Work out the finished part from the listing and answer in its coordinate system (mm). Face numbers are marked on the shaded views. A direction names the side the tool comes from. Coordinates: 2 decimals unless noted, no trailing zeros. Order: outer loops, then holes, each group sorted by start corner. A loop starts at its lowest first (then second) coordinate and runs counter-clockwise, first axis right, second up. Notation, with made-up numbers: (-9, 1) -> (9, 1) arc R32 cw to (9, 29) -> close; hole circle Ø11 at (-18.75, -0.75). An arc over 180 degrees is marked (long way). Answer as CSV lines item,"result". Start each with the question number.
Item 1: A straight line is drawn through the part: L1, parallel to X at y = 12, z = 96 (3 decimals). Find the intervals that lie inside material, in ascending order.
Item 2: Section D-D (y = 45) is taken. Write down the section's boundary in (x, z) (3 decimals).
Item 3: Section A-A (y = 19.05) is taken. Write down the section's boundary in (x, z) (1 decimal).
Item 4: Section C-C (z = 145) is taken. Write down the section's boundary in (x, y) (3 decimals), then the cut area to 3 significant figures.
Item 5: Each of these flat-tipped pins is pushed along its axis until it touches: pin 1 Ø2 at (y, z) = (45, 113.5) entering from +X (3 decimals); pin 2 Ø2.5 at (x, y) = (15, 2) entering from -Z (3 decimals); pin 3 Ø1.6 at (x, z) = (1, 467.5) entering from -Y (3 decimals); pin 4 Ø12 at (x, y) = (11.5, 39) entering from +Z. Where does it stop, or does it pass through?
Item 6: Section B-B (x = 8.5) is taken. Write down the section's boundary in (y, z) (3 decimals).
Item 7: Which of the six approach directions +Z, -Z, +X, -X, +Y, -Y give full straight-line access (tool end or side, diameter ignored) to the marked faces 1 and 2?
Autodesk Inventor part; units mm, degrees
ref_plane "YZ Plane" through (0, 0, 0) normal (1, 0, 0) x (0, 1, 0)
ref_plane "XZ Plane" through (0, 0, 0) normal (0, 1, 0) x (-1, 0, 0)
ref_plane "XY Plane" through (0, 0, 0) normal (0, 0, 1) x (1, 0, 0)
sketch "Sketch1" plane through (0, 0, 0) normal (0, 0, 1) x (1, 0, 0)
  line L0 (0, 0) -> (25.4, 0)
  line L1 (25.4, 0) -> (25.4, 3.175)
  line L2 (3.175, 50.8) -> (0, 50.8)
  line L3 (0, 50.8) -> (0, 0)
  line L4 (3.175, 50.8) -> (3.175, 3.175)
  line L5 (3.175, 3.175) -> (25.4, 3.175)
  dimension "d0" = 50.8
  dimension "d1" = 25.4
  dimension "d2" = 3.175
  dimension "d3" = 3.175
extrude "Extrusion1" add sketch "Sketch1" along normal blind 482.6
sketch "Sketch2" plane through (0, 0, 0) normal (-1, 0, 0) x (0, 0, 1)
  line L0 (482.6, 0) -> (482.6, 50.8)
  line L1 (0, 0) -> (482.6, 0)
  circle A0 centre (466.725, 19.05) radius 11.1125
  dimension "d6" = 22.225
  dimension "d7" = 19.05
  dimension "d8" = 15.875
extrude "Extrusion2" cut sketch "Sketch2" against normal blind 508
sketch "Sketch3" plane through (0, 0, 0) normal (0, -1, 0) x (1, 0, 0)
  line L0 (0, 0) -> (0, 482.6)
  line L1 (0, 0) -> (25.4, 0)
  line L2 (25.4, 0) -> (25.4, 482.6)
  line L3 (0, 22.225) -> (25.4, 22.225)
  line L4 (25.4, 482.6) -> (0, 482.6)
  line L5 (0, 460.375) -> (25.4, 460.375)
  dimension "d13" = 22.225
  dimension "d16" = 22.225
extrude "Extrusion3" cut sketch "Sketch3" against normal blind 3.175 contours L0 L3 L2 L1 | L0 L4 L2 L5
equation "\"d3\" = d2"
equation "\"d16\" = d13"
properties part number "manipulator L frame right"
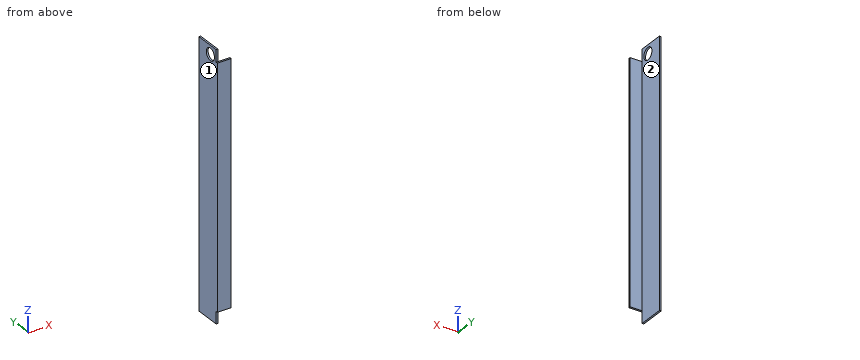
Checked values:
1,L1,"x = 0 to 3.175"
2,outline,"(0, 0) -> (3.175, 0) -> (3.175, 482.6) -> (0, 482.6) -> close"
3,outline,"(0, 0) -> (3.2, 0) -> (3.2, 455.6) -> (0, 455.6) -> close; (0, 477.8) -> (3.2, 477.8) -> (3.2, 482.6) -> (0, 482.6) -> close"
4,outline,"(0, 0) -> (25.4, 0) -> (25.4, 3.175) -> (3.175, 3.175) -> (3.175, 50.8) -> (0, 50.8) -> close"
4,area,"232 mm^2"
5,pin 1,"stops at x = 3.175"
5,pin 2,"stops at z = 22.225"
5,pin 3,"stops at y = 3.175"
5,pin 4,"passes through"
6,outline,"(0, 22.225) -> (3.175, 22.225) -> (3.175, 460.375) -> (0, 460.375) -> close"
7,face 1,"+Z, -Z, -X, +Y, -Y"
7,face 2,"+Z, -Z, +X, +Y"
